```python
from build123d import *

# Parameters (mm, degrees)
CUT_EXTRUDE1_DEPTH = 2.5


with BuildPart() as part:
    # Sketch1 → Revolve1 (revolve)
    with BuildSketch(Plane.XY, mode=Mode.PRIVATE) as revolve1_sk:
        Polygon((-64, 7.5), (-64, 0), (68, 0), (68, 7.5), (4, 7.5), (4, 12.5), (-4, 12.5), (-4, 7.5), align=None)
        with BuildLine():
            Line((69.770509831, 0), (68, 0))
            Line((68, 0), (68, 7.5))
            ThreePointArc((68, 7.5), (69.321881746, 3.853073613), (69.770509831, 0))
        make_face()
        with BuildLine():
            Line((-64, 0), (-64, 7.5))
            ThreePointArc((-64, 7.5), (-65.321881746, 3.853073613), (-65.770509831, 0))
            Line((-65.770509831, 0), (-64, 0))
        make_face()
    revolve(revolve1_sk.sketch.rotate(Axis((-80.68485448, 0, 0), (1, 0, 0)), 90), axis=Axis((-80.68485448, 0, 0), (1, 0, 0)))

    # Sketch2 → Cut-Extrude1 (cut, symmetric)
    with BuildSketch(Plane.XY):
        Polygon((51, 10), (51, 5), (16, 5), (16, 9.65), align=None)
    extrude(amount=CUT_EXTRUDE1_DEPTH, both=True, mode=Mode.SUBTRACT)


solid = part.part
```
Work out the finished part from the listing and answer in its coordinate system (mm). A direction names the side the tool comes from. Coordinates: 2 decimals unless noted, no trailing zeros. Write each loop counter-clockwise with the first axis right and the second up, starting at its lowest first coordinate (ties: lowest second). Pieces come first, ordered by that corner, then holes.
Q1. A cutting plane is placed at B-B, the plane z = 4. Give the vertices of the cut face in (x, y), then the cut area to 3 significant figures.
Q2. Determine the mould class of faces 5 (the face through (-34.42, -6.324, 4.032)), 6 (the face through (51, 6, 0)), 7 (the face through (4, 8, 0)) for opening direction X: released by +X, released by -X, zero draft, split by the parting line, or undercut.
Q3. A cutting plane is placed at C-C, the plane x = 58. Give the vertices of the cut face in (y, z), then the cut area to 3 significant figures.
Q4. A cutting plane is placed at A-A, the plane y = 0. Give the vertices of the cut face in (x, z), then the cut area to 3 significant figures.
Q5. A cutting plane is placed at D-D, the plane x = 41.5. Give the vertices of the cut face in (y, z), then the cut area to 3 significant figures.
Q6. Each of these flat-tipped pins is pushed along its axis until it touches: pin 1 Ø1 at (x, y) = (13, -2) entering from +Z; pin 2 Ø2 at (y, z) = (7, -1) entering from -X; pin 3 Ø2 at (x, y) = (-23, -3.5) entering from +Z. Where does it stop, or does it pass through?
Q7. Which of the six approach directions +Z, -Z, +X, -X, +Y, -Y give full straight-line access (tool end or side, diameter ignored) to faces 1 (the face through (16, 6, 0)), 2 (the face through (35.552, -6.324, 4.032)), 3 (the face through (-0.056, -3.755, 11.923)), 4 (the face through (-4, 8, 0))?
Q8. Find the intervals of material crossed by line 1 (X direction, y = 10.5, z = 6); line 2 (Y direction, x = 8.5, z = -3.5); line 3 (Y direction, x = 19, z = 5), in increasing order.
Findings below:
1. outline: (-64, -6.34) - (-4, -6.34) - (-4, -11.84) - (4, -11.84) - (4, -6.34) - (68, -6.34) arc R16.29 ccw to (68, 6.34) - (4, 6.34) - (4, 11.84) - (-4, 11.84) - (-4, 6.34) - (-64, 6.34) arc R16.29 ccw to start
1. area: 1,780 mm2
2. face 5: zero draft
2. face 6: undercut
2. face 7: released by +X
3. outline: circle Ø15 at (0, 0)
3. area: 177 mm2
4. outline: (-64, -7.5) - (-4, -7.5) - (-4, -12.5) - (4, -12.5) - (4, -7.5) - (68, -7.5) arc R16.77 ccw to (68, 7.5) - (4, 7.5) - (4, 12.5) - (-4, 12.5) - (-4, 7.5) - (-64, 7.5) arc R16.77 ccw to start
4. area: 2,100 mm2
5. outline: (5, -2.5) - (5, 2.5) - (7.07, 2.5) arc R7.5 ccw (long way) to (7.07, -2.5) - close
5. area: 165 mm2
6. pin 1: stops at z = 7.35
6. pin 2: stops at x = -64.63
6. pin 3: stops at z = 7.07
7. face 1: +Y
7. face 2: +X
7. face 3: +X, -X
7. face 4: -X
8. line 1: x = -4 to 4
8. line 2: y = -6.63 to 6.63
8. line 3: y = -5.59 to 5.59
